CAD build for the part. Positions are in the model's coordinates, mm. Face numbers are marked on the shaded views. A direction names the side the tool comes from. Coordinates: 2 decimals unless noted, no trailing zeros. Loops run counter-clockwise (first coordinate to the right, second up) from the corner with the lowest first, then second, coordinate; pieces in that order, holes last.
1) Wall check: line 1 along Y through (x, z) = (-67.5, -0.5); line 2 along Z through (x, y) = (-56.5, -8.75); line 3 along X through (y, z) = (-9, -2.5). Give the ranges that are in metal, low to high.
2) Saw through at D-D, the plane x = -53.5. Write the cut outline in (y, z), and give its area (3 significant figures).
3) Saw through at A-A, the plane z = -0.75. Write the cut outline in (x, y), and give its area (3 significant figures).
4) Saw through at B-B, the plane x = -67.5. Write the cut outline in (y, z), and give its area (3 significant figures).
5) Saw through at C-C, the plane y = -7.25. Write the cut outline in (x, z), and give its area (3 significant figures).
6) Which spindle directions (+Z, -Z, +X, -X, +Y, -Y) get a long thin tool onto all of the face, cutting with end or side? Do the marked faces 5, 6, 7, 8 and 9. Say none if no direction does.
7) Pin check, flat tips, straight feed: pin 1 Ø4 at (y, z) = (-9, -3) entering from +X; pin 2 Ø1.1 at (x, z) = (-71, -2.5) entering from +Y; pin 3 Ø4 at (x, y) = (-53.5, -8) entering from -Z; pin 4 Ø4 at (x, y) = (-73, -6) entering from -Z. Stop position of each tip, or through.
8) Two-plate mould, pull along X, no slides. Class the marked faces 1, 2, 3 and 4: +X half, -X half, draft (parallel to the pull), parting line (faces both ways), or undercut.
```python
from build123d import *

# Parameters (mm, degrees)
SKETCH_1_R       = 2.45
EXTRUDE_1_DEPTH  = 2
SKETCH_1_3_R     = 2.45
EXTRUDE_2_DEPTH  = 2
SKETCH_3_W       = 2.5
SKETCH_3_H       = 4.5
EXTRUDE_3_DEPTH  = 2
SKETCH_5_R       = 2.45
EXTRUDE_4_DEPTH  = 5
EXTRUDE_8_DEPTH  = 2
SKETCH_13_W      = 2
SKETCH_13_H      = 3
EXTRUDE_12_DEPTH = 1
SKETCH_16_R      = 2.45
EXTRUDE_16_DEPTH = 5


with BuildPart() as part:
    # Sketch 1 → Extrude 1 (new body)
    with BuildSketch(Plane.XY):
        with BuildLine():
            Line((-56.860741066, -7.81033927), (-60.460741066, -7.81033927))
            Line((-60.460741066, -7.81033927), (-60.460741066, -3.31033927))
            Line((-60.460741066, -3.31033927), (-52.360741066, -3.31033927))
            ThreePointArc((-52.360741066, -3.31033927), (-49.178760551, -10.992319786), (-56.860741066, -7.81033927))
        make_face()
        with Locations((-52.360741066, -7.81033927)):
            Circle(SKETCH_1_R, mode=Mode.SUBTRACT)
    extrude(amount=EXTRUDE_1_DEPTH)



with BuildPart() as body_2:
    # Sketch 1_3 → Extrude 2 (new body)
    with BuildSketch(Plane.XY):
        with BuildLine():
            Line((-72.411189037, -12.31033927), (-70.458584645, -12.31033927))
            Line((-70.458584645, -12.31033927), (-70.458584645, -13.81033927))
            Line((-70.458584645, -13.81033927), (-65.458584645, -13.81033927))
            Line((-65.458584645, -13.81033927), (-60.458584645, -13.81033927))
            Line((-60.458584645, -13.81033927), (-60.460741066, -12.31033927))
            Line((-60.460741066, -12.31033927), (-60.460741066, -7.81033927))
            Line((-60.460741066, -7.81033927), (-60.460741066, -3.31033927))
            Line((-60.460741066, -3.31033927), (-78.460741066, -3.31033927))
            ThreePointArc((-78.460741066, -3.31033927), (-82.960741066, -7.81033927), (-78.460741066, -12.31033927))
            Line((-78.460741066, -12.31033927), (-72.411189037, -12.31033927))
        make_face()
        with Locations((-78.460741066, -7.81033927)):
            Circle(SKETCH_1_3_R, mode=Mode.SUBTRACT)
    extrude(amount=-EXTRUDE_2_DEPTH)


with BuildPart() as part_1:
    add(part.part)

    add(body_2.part)  # Extrude 3 merges body 2
    # Sketch 3 → Extrude 3 (add)
    with BuildSketch(Plane.XY):
        with Locations((-61.710741066, -5.56033927)):
            Rectangle(SKETCH_3_W, SKETCH_3_H)
    extrude(amount=EXTRUDE_3_DEPTH)

    # Sketch 5 → Extrude 4 (add)
    with BuildSketch(Plane.XY.offset(2)):
        with Locations((-52.360741066, -7.81033927)):
            Circle(SKETCH_5_R)
    extrude(amount=-EXTRUDE_4_DEPTH)

    # Sketch 10 → Extrude 8 (add)
    with BuildSketch(Plane(origin=(0, 0, -2), x_dir=(-1, 0, 0), z_dir=(0, 0, -1))):
        Polygon((70.458584645, -12.31033927), (71.458584645, -12.31033927), (71.458584645, -13.81033927), (71.458584645, -15.91033927), (70.458584645, -15.91033927), (60.458584645, -15.91033927), (60.458584645, -14.91033927), (70.458584645, -14.91033927), (70.458584645, -13.81033927), align=None)
    extrude(amount=-EXTRUDE_8_DEPTH)

    # Sketch 13 → Extrude 12 (add)
    with BuildSketch(Plane(origin=(0, 0, -2), x_dir=(-1, 0, 0), z_dir=(0, 0, -1))):
        with Locations((70.458584645, -14.41033927)):
            Rectangle(SKETCH_13_W, SKETCH_13_H)
    extrude(amount=EXTRUDE_12_DEPTH)

    # Sketch 16 → Extrude 16 (add)
    with BuildSketch(Plane.XY):
        with Locations((-78.460741066, -7.81033927)):
            Circle(SKETCH_16_R)
    extrude(amount=-EXTRUDE_16_DEPTH)


solid = part_1.part
```
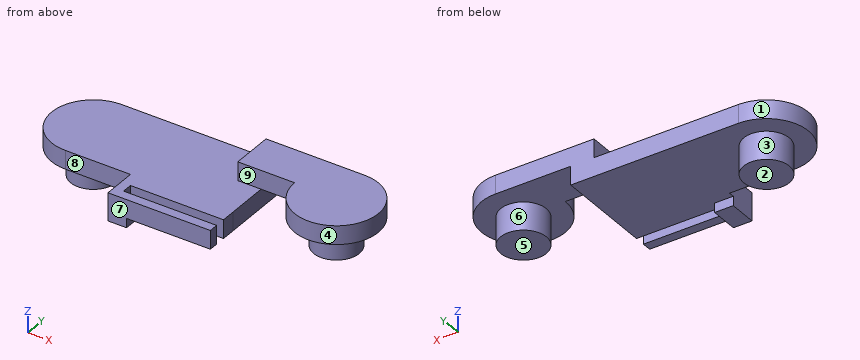
Data:
1. line 1: y = -15.91 to -14.91, -13.81 to -3.31
1. line 2: z = 0 to 2
1. line 3: x = -80.6 to -76.32, -54.5 to -50.22
2. outline: (-12.16, 0) - (-9.98, 0) - (-9.98, -3) - (-5.64, -3) - (-5.64, 0) - (-3.31, 0) - (-3.31, 2) - (-12.16, 2) - close
2. area: 30.7 mm2
3. outline: (-78.46, -12.31) - (-71.46, -12.31) - (-71.46, -15.91) - (-60.46, -15.91) - (-60.46, -14.91) - (-70.46, -14.91) - (-70.46, -13.81) - (-60.46, -13.81) - (-60.46, -12.31) - (-60.46, -3.31) - (-78.46, -3.31) arc R4.5 ccw to start; circle Ø4.9 at (-52.36, -7.81)
3. area: 241 mm2
4. outline: (-15.91, -2) - (-14.91, -2) - (-14.91, 0) - (-15.91, 0) - close; (-13.81, -2) - (-3.31, -2) - (-3.31, 0) - (-13.81, 0) - close
4. area: 23.0 mm2
5. outline: (-82.93, -2) - (-80.85, -2) - (-80.85, -5) - (-76.08, -5) - (-76.08, -2) - (-60.46, -2) - (-60.46, 0) - (-54.75, 0) - (-54.75, -3) - (-49.98, -3) - (-49.98, 0) - (-47.9, 0) - (-47.9, 2) - (-62.96, 2) - (-62.96, 0) - (-82.93, 0) - close
5. area: 104 mm2
6. face 5: -Z, +X, +Y, -Y
6. face 6: -Z
6. face 7: +Z, -Z, +X, -X, -Y
6. face 8: +Z, -Z, -X, -Y
6. face 9: +Z, -X, -Y
7. pin 1: stops at x = -49.91
7. pin 2: stops at y = -3.31
7. pin 3: stops at z = -3
7. pin 4: stops at z = -2
8. face 1: -X half
8. face 2: draft
8. face 3: undercut
8. face 4: parting line
